Geometry: see drawing. Coordinates: mm, zero at the bounding-box minimum. A direction names the side the tool comes from. Round coordinates to 2 decimals unless told otherwise and drop trailing zeros. Write each loop counter-clockwise with the first axis right and the second up, starting at its lowest first coordinate (ties: lowest second). Pieces come first, ordered by that corner, then holes. Notation, with made-up numbers: (47.5, 87.25) -> (71.5, 87.25) arc R36 cw to (71.5, 122.25) -> close; hole circle Ø4 at (-24, 62.5). An arc over 180 degrees is marked (long way). Use CSV: the item, a comma, the result in double quotes.
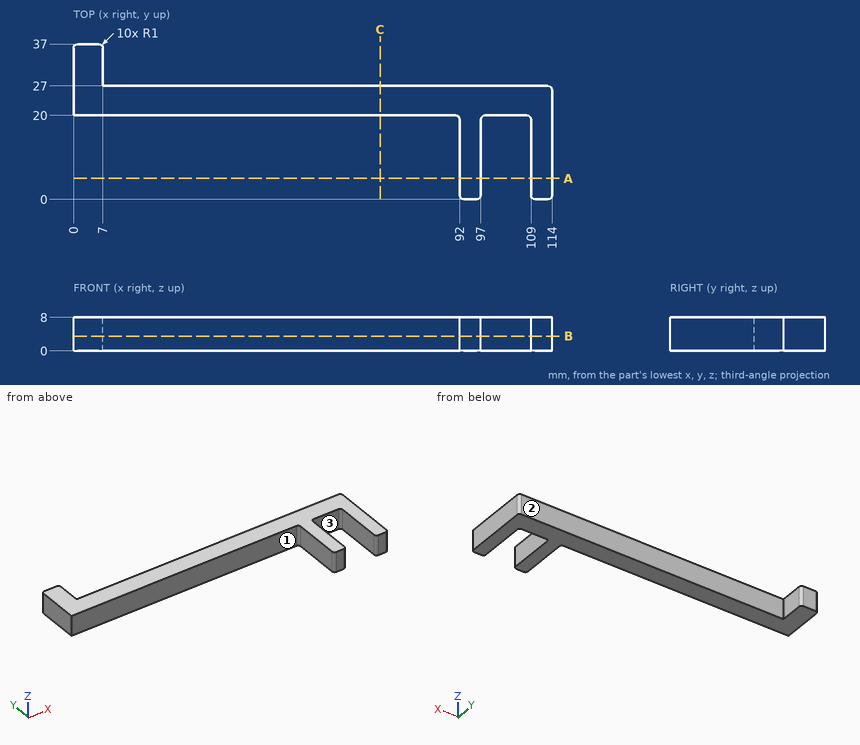
Item 1: Section query C-C on x = 73. Return the cut outline in (y, z), plus the area to 3 significant figures.
Worked answers:
outline,"(20, 0) -> (27, 0) -> (27, 8) -> (20, 8) -> close"
area,"56.0 mm²"
Item 2: Set-up query: the marked faces 1, 2 and 3. Return all of +Z, -Z, +X, -X, +Y, -Y with unobstructed straight access to the full face (end or side cutting, diameter ignored); none if empty.
Worked answers:
face 1,"+Z, -Z, -X, -Y"
face 2,"+Z, -Z, +X, +Y"
face 3,"+Z, -Z, -Y"
Item 3: First-contact query: pin 1 Ø2 at (y, z) = (12, 6.5) entering from -X; pin 2 Ø4 at (x, z) = (47.5, 4) entering from +Y; pin 3 Ø2.5 at (x, z) = (27.5, 5) entering from -Y. Flat tips, straight axial feed; report the tip coordinate or a pass-through.
Worked answers:
pin 1,"stops at x = 92"
pin 2,"stops at y = 27"
pin 3,"stops at y = 20"
Item 4: Section query B-B on z = 3.5. Return the cut outline in (x, y).
Worked answers:
outline,"(0, 20) -> (91, 20) arc R1 cw to (92, 19) -> (92, 1) arc R1 ccw to (93, 0) -> (96, 0) arc R1 ccw to (97, 1) -> (97, 19) arc R1 cw to (98, 20) -> (108, 20) arc R1 cw to (109, 19) -> (109, 1) arc R1 ccw to (110, 0) -> (113, 0) arc R1 ccw to (114, 1) -> (114, 26) arc R1 ccw to (113, 27) -> (7, 27) -> (7, 36) arc R1 ccw to (6, 37) -> (1, 37) arc R1 ccw to (0, 36) -> close"
Item 5: Section query A-A on y = 5. Return the cut outline in (x, z).
Worked answers:
outline,"(92, 0) -> (97, 0) -> (97, 8) -> (92, 8) -> close; (109, 0) -> (114, 0) -> (114, 8) -> (109, 8) -> close"
Item 6: Line query: line 1 (X direction, y = 3, z = 2.75); line 2 (Y direction, x = 46.5, z = 4); line 3 (X direction, y = 32.5, z = 1). Output: solid intervals per line, ascending.
Worked answers:
line 1,"x = 92 to 97, 109 to 114"
line 2,"y = 20 to 27"
line 3,"x = 0 to 7"
